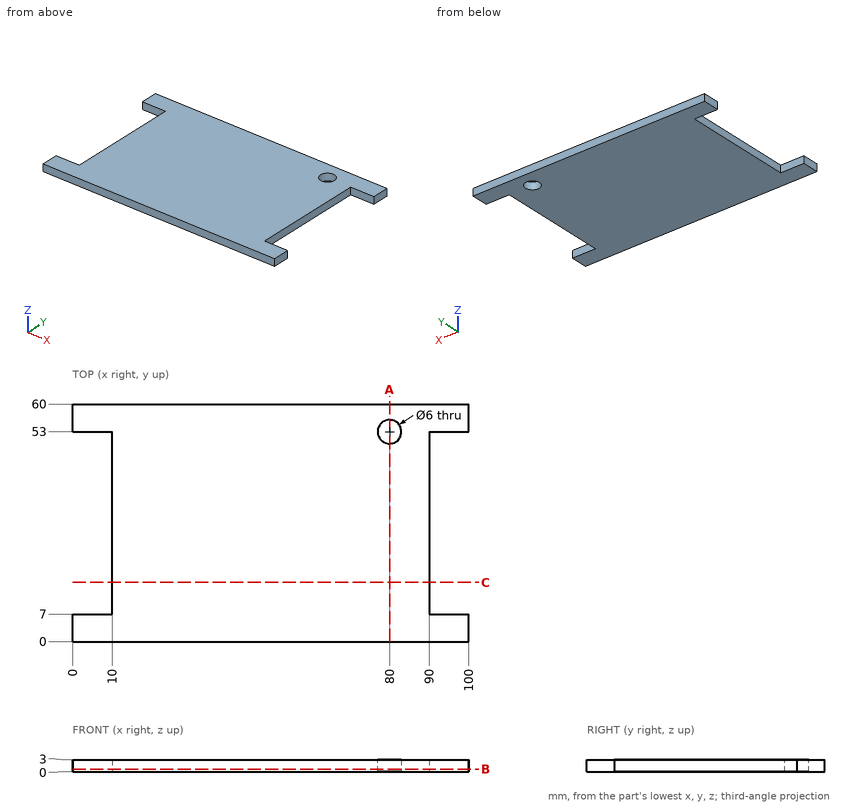
Source: three-view drawing plus pictorial views. Frame: mm from the lowest corner of the part. Give positions to 0.01 mm unless a question says otherwise; leave off trailing zeros. Order: outer loops, then holes, each group sorted by start corner. A loop starts at its lowest first (then second) coordinate and runs counter-clockwise, first axis right, second up. Notation, with made-up numbers: (78, 34.5) -> (125, 34.5) arc R20 ccw to (125, 39.5) -> close; hole circle Ø9 at (57, 70). An arc over 180 degrees is marked (long way). Write each question's results on one line, items separated by ' | '. Start each with the question number.
Item 1: Cut plane B-B on z = 0.65. Return the cut outline in (x, y).
Item 2: Cut plane A-A on x = 80. Return the cut outline in (y, z).
Item 3: Cut plane C-C on y = 15. Return the cut outline in (x, z), then the cut area to 3 significant figures.
Item 4: Contact query for a flat-ended pin moving along its axis: P1, Ø1.5, axis at y = 20, z = 1.5, coming from the +X side. Output: stop coordinate, or through.
Item 5: Line query: line 1 (Y direction, x = 80, z = 1.5); line 2 (Y direction, x = 91, z = 2.25); line 3 (X direction, y = 43, z = 2.6). Output: solid intervals per line, ascending.
Established:
1) outline: (0, 0) -> (100, 0) -> (100, 7) -> (90, 7) -> (90, 53) -> (100, 53) -> (100, 60) -> (0, 60) -> (0, 53) -> (10, 53) -> (10, 7) -> (0, 7) -> close; hole circle Ø6 at (80, 53)
2) outline: (0, 0) -> (50, 0) -> (50, 3) -> (0, 3) -> close; (56, 0) -> (60, 0) -> (60, 3) -> (56, 3) -> close
3) outline: (10, 0) -> (90, 0) -> (90, 3) -> (10, 3) -> close | area: 240 mm^2
4) P1: x = 90
5) line 1: 0 to 50, 56 to 60 | line 2: 0 to 7, 53 to 60 | line 3: 10 to 90
